Check sheet for the drawn part. Datum: minimum x, y, z corner. Units: mm. Round coordinates to 2 decimals unless told otherwise and drop trailing zeros. Write each loop counter-clockwise with the first axis right and the second up, starting at its lowest first coordinate (ties: lowest second). Pieces come first, ordered by that corner, then holes.
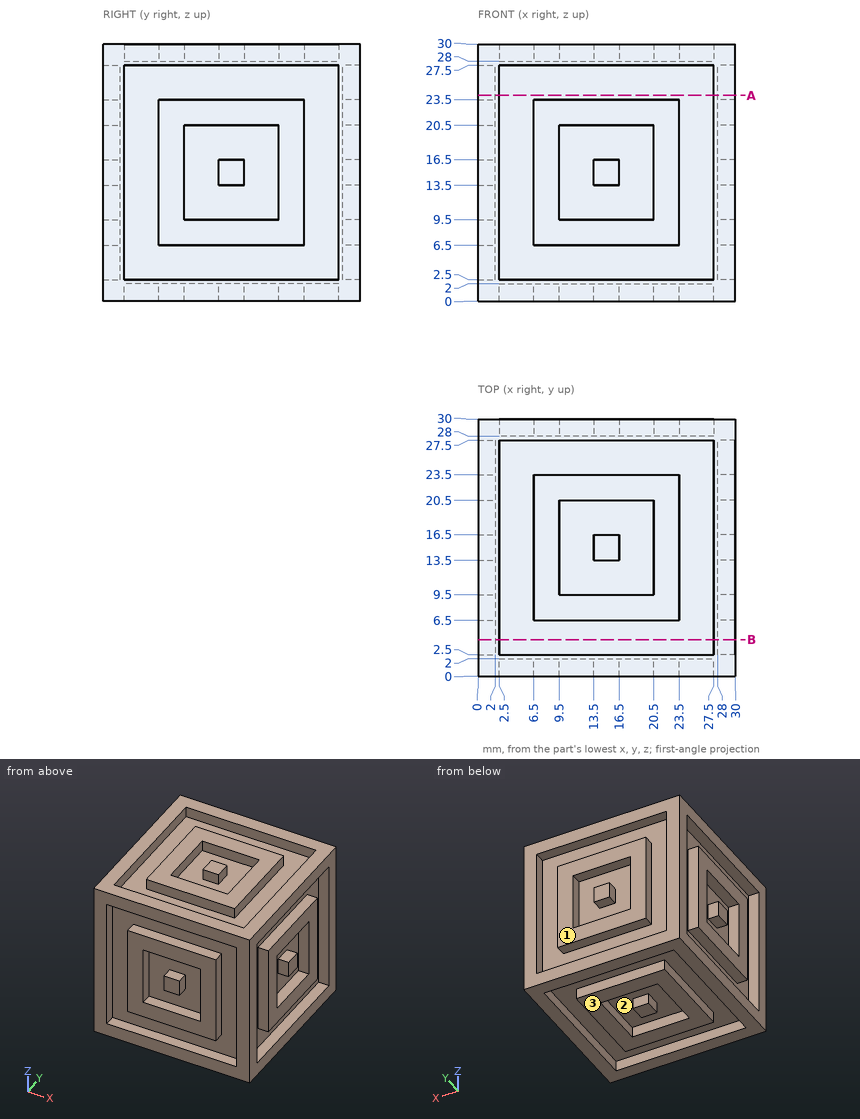
Q1. Material ranges on line 1 along Z through (x, y) = (7, 28.25); line 2 along Y through (x, z) = (3, 28.75); line 3 along Y through (x, z) = (9.75, 1.75), recorded low to high.
Recorded:
line 1: z = 0 to 2.5, 6.5 to 23.5, 27.5 to 30
line 2: y = 0 to 2.5, 27.5 to 30
line 3: y = 0 to 2.5, 6.5 to 9.5, 20.5 to 23.5, 27.5 to 30
Q2. Release check for a two-part mould opening along Y. For the marked faces 1, 2 and 3 record: released by +Y, released by -Y, zero draft, split by the parting line, or undercut.
Recorded:
face 1: released by +Y
face 2: undercut
face 3: zero draft
Q3. Depth check by flat-ended pin: P1, Ø1.5, axis at x = 24.5, y = 25, coming from the +Z side. Enter the tip coordinate at first touch or a pass-through.
Recorded:
P1: stops at z = 28
Q4. Sectioned sample at A-A (z = 24). Enter the section's corners in (x, y).
Recorded:
outline: (0, 0) - (2.5, 0) - (2.5, 2) - (27.5, 2) - (27.5, 0) - (30, 0) - (30, 2.5) - (28, 2.5) - (28, 27.5) - (30, 27.5) - (30, 30) - (27.5, 30) - (27.5, 28) - (2.5, 28) - (2.5, 30) - (0, 30) - (0, 27.5) - (2, 27.5) - (2, 2.5) - (0, 2.5) - close
